Autodesk Inventor part; units mm, degrees
ref_plane "Work Plane2" through (0, 0, -38.1) normal (0, 0, 1) x (1, 0, 0)
ref_plane "YZ Plane" through (0, 0, 0) normal (1, 0, 0) x (0, 1, 0)
ref_plane "XZ Plane" through (0, 0, 0) normal (0, 1, 0) x (-1, 0, 0)
sketch "Sketch1" plane through (0, 0, 0) normal (0, 1, 0) x (-1, 0, 0)
  circle A0 centre (0, 0) radius 50.8
  dimension "d0" = 101.6
extrude "Extrusion1" add sketch "Sketch1" along normal blind 24
ref_plane "Work Plane1" through (0, 0, 50.8) normal (0, 0, 1) x (1, 0, 0)
sketch "Sketch3" plane through (0, 0, 50.8) normal (0, 0, 1) x (1, 0, 0)
  line L0 (50.8, 24) -> (-50.8, 24)
  line L1 (0, 24) -> (0, 12) construction
  point P0 (0, 0)
  dimension "d7" = 12
hole "Hole1" at (0, 12, 50.8) direction (0, 0, -1) diameter 16.5 depth 88.9 tip angle 118
sketch "Sketch4" plane through (0, 0, 0) normal (0, -1, 0) x (1, 0, 0)
  line L0 (0, 0) -> (0, -25) construction
  line L1 (0, 0) -> (0, 25) construction
  dimension "d15" = 25
  dimension "d16" = 25
hole "Hole2" at (0, 0, 25) at (0, 0, -25) direction (0, 1, 0) diameter 4.134 end up to surface
sketch "Sketch5" plane through (0, 0, 0) normal (0, -1, 0) x (1, 0, 0)
  point P0 (0, 0)
  point P1 (-19.6272, 0)
hole "Hole3" at (-19.6272, 0, 0) direction (0, 1, 0) diameter 4.917 depth 12 tip angle 118
ref_plane "Work Plane2" through (0, 0, -38.1) normal (0, 0, 1) x (1, 0, 0)
sketch "Sketch7" plane through (0, 24, 0) normal (0, 1, 0) x (1, 0, 0)
  circle A0 centre (0, 0) radius 50.8
  circle A1 centre (0, 0) radius 47.5
  dimension "d35" = 101.6
  dimension "d36" = 95
extrude "Extrusion4" cut sketch "Sketch7" against normal blind 1
properties part number "Platogrueso" material "Aluminum 6061"
Work out the finished part from the listing and answer in its coordinate system (mm). A direction names the side the tool comes from. Give positions to 0.01 mm unless a question says otherwise; leave off trailing zeros. Order: outer loops, then holes, each group sorted by start corner. A loop starts at its lowest first (then second) coordinate and runs counter-clockwise, first axis right, second up. Notation, with made-up numbers: (86.25, -25.5) - (124.25, -25.5) arc R16 ccw to (124.25, -21.5) - close; hole circle Ø5 at (51, 21.25). An arc over 180 degrees is marked (long way). Answer as CSV lines item,"result". Start each with the question number.
Q1. Find the intervals of material crossed by L1, parallel to Z at x = 0, y = 1.1; L2, parallel to Y at x = 0, z = -11; L3, parallel to X at y = 10, z = 14, in increasing order. Write a range as [from, to].
Q2. The part is cut by section C-C (z = -25). Write down the section's boundary in (x, y), then the cut area to 3 significant figures.
Q3. The mould has two halves that part along Z. Classify faces 6 (the face through (-20.01, 13.22, -0.2)), 7 (the face through (34, 23, 34)), 8 (the face through (11.012, 11.339, 49.592)), 9 (the face through (-0.091, 2.035, 27.065)): +Z half, -Z half, draft (parallel to the pull), parting line (faces both ways), or undercut.
Q4. The part is cut by section A-A (z = -7.5). Write down the section's boundary in (x, y), then the cut area to 3 significant figures.
Q5. The part is cut by section B-B (x = -40.5). Write down the section's boundary in (y, z), then the cut area to 3 significant figures.
Q6. Given pin 1 Ø2 at (y, z) = (6.5, -35) entering from -X; pin 2 Ø5 at (y, z) = (5.5, 23) entering from -X; pin 3 Ø4 at (x, y) = (-12.5, 4.5) entering from +Z, each flat-ended and moving along its own axis, determine where each tip first touches the part or whether it passes through.
Q7. The part is cut by section D-D (z = -36). Write down the section's boundary in (x, y).
Q8. For faces 1 (the face through (1, 0, 1)), 2 (the face through (-10.3, 23.51, 46.37)), 3 (the face through (-2.48, 4.13, 5.73)), 4 (the face through (1, 24, 1)), 5 (the face through (-0.091, 2.035, -22.935)), determine the directions among +Z, -Z, +X, -X, +Y, -Y from which every point of the face is accessible in a straight line to the end or side of a thin tool.
Check result:
1,L1,"z = [-50.8, -27.07], [-22.93, 22.93], [27.07, 50.8]"
1,L2,"y = [0, 3.75], [20.25, 24]"
1,L3,"x = [-48.83, -8], [8, 48.83]"
2,outline,"(-44.22, 0) - (-2.07, 0) - (-2.07, 4.01) arc R8.25 cw (long way) to (2.07, 4.01) - (2.07, 0) - (44.22, 0) - (44.22, 23) - (40.39, 23) - (40.39, 24) - (-40.39, 24) - (-40.39, 23) - (-44.22, 23) - close"
2,area,"1,890 mm²"
3,face 6,"undercut"
3,face 7,"draft"
3,face 8,"parting line"
3,face 9,"undercut"
4,outline,"(-50.24, 0) - (50.24, 0) - (50.24, 23) - (46.9, 23) - (46.9, 24) - (-46.9, 24) - (-46.9, 23) - (-50.24, 23) - close; hole circle Ø16.5 at (0, 12)"
4,area,"2,190 mm²"
5,outline,"(0, -30.67) - (23, -30.67) - (23, -24.82) - (24, -24.82) - (24, 24.82) - (23, 24.82) - (23, 30.67) - (0, 30.67) - close"
5,area,"1,460 mm²"
6,pin 1,"stops at x = -37.74"
6,pin 2,"stops at x = -46.48"
6,pin 3,"stops at z = 49.7"
7,outline,"(-35.84, 0) - (35.84, 0) - (35.84, 23) - (30.99, 23) - (30.99, 24) - (-30.99, 24) - (-30.99, 23) - (-35.84, 23) - close; hole circle Ø16.5 at (0, 12)"
8,face 1,"+Z, -Z, +X, -X, -Y"
8,face 2,"+Y"
8,face 3,"+Z"
8,face 4,"+Z, -Z, +X, -X, +Y"
8,face 5,"-Y"
